Model file for the job. Use its own axes, mm. Face numbers are marked on the shaded views. A direction names the side the tool comes from. Round coordinates to 2 decimals unless told otherwise and drop trailing zeros. One line per item, written item: value.
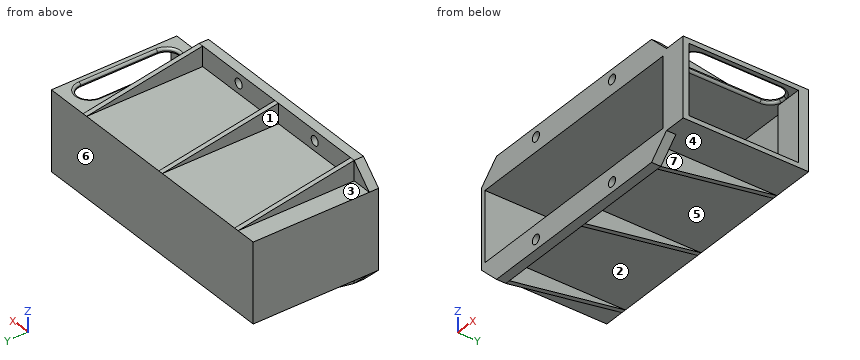
from build123d import *

# Parameters (mm, degrees)
SKETCH1_W                 = 166.85
SKETCH1_H                 = 54.05
SKETCH1_W_2               = 160.5
SKETCH1_H_2               = 47.7
BOSS_EXTRUDE1_DEPTH       = 3.81
BOSS_EXTRUDE2_DEPTH       = 78.232
SKETCH3_W                 = 166.85
SKETCH3_H                 = 54.05
BOSS_EXTRUDE5_DEPTH       = 3.175
SKETCH4_W                 = 3.175
SKETCH4_H                 = 54.05
BOSS_EXTRUDE6_DEPTH       = 3.81
BOSS_EXTRUDE7_DEPTH       = 6.35
BOSS_EXTRUDE9_DEPTH       = 3.175
BOSS_EXTRUDE10_DEPTH      = 3.175
SKETCH8_R                 = 3.175
CUT_EXTRUDE1_DEPTH        = 122.77066278
BOSS_EXTRUDE11_DEPTH      = 1.5875
BOSS_EXTRUDE11_DEPTH_BACK = 1.5875
SKETCH14_W                = 54.05
SKETCH14_H                = 85.217
SKETCH14_W_2              = 47.7
SKETCH14_H_2              = 74.422
BOSS_EXTRUDE13_DEPTH      = 14.986
CUT_EXTRUDE2_DEPTH        = 147.696293869
SKETCH16_W                = 160.5
SKETCH16_H                = 47.7
CUT_EXTRUDE3_DEPTH        = 1.5875
SKETCH17_W                = 18.712657602
SKETCH17_H                = 69.277031054
BOSS_EXTRUDE14_DEPTH      = 3.175
FILLET1_R                 = 1.5875


with BuildPart() as part:
    # Sketch1 → Boss-Extrude1 (new body)
    with BuildSketch(Plane(origin=(0, 0, 0), x_dir=(1, 0, 0), z_dir=(0, 1, 0))):
        Rectangle(SKETCH1_W, SKETCH1_H)
        Rectangle(SKETCH1_W_2, SKETCH1_H_2, mode=Mode.SUBTRACT)
    extrude(amount=BOSS_EXTRUDE1_DEPTH)

    # Sketch2 → Boss-Extrude2 (add)
    with BuildSketch(Plane(origin=(0, 3.81, 0), x_dir=(1, 0, 0), z_dir=(0, 1, 0))):
        Polygon((-83.425, 27.025), (83.425, 27.025), (83.425, 23.85), (80.25, 23.85), (-80.25, 23.85), (-80.25, -23.85), (80.25, -23.85), (83.425, -23.85), (83.425, -27.025), (-83.425, -27.025), align=None)
    extrude(amount=BOSS_EXTRUDE2_DEPTH)

    # Sketch3 → Boss-Extrude5 (add)
    with BuildSketch(Plane(origin=(0, 82.042, 0), x_dir=(1, 0, 0), z_dir=(0, 1, 0))):
        Rectangle(SKETCH3_W, SKETCH3_H)
    extrude(amount=BOSS_EXTRUDE5_DEPTH)

    # Sketch4 → Boss-Extrude6 (add)
    with BuildSketch(Plane.XZ.offset(-82.042)):
        with Locations((81.8375, 0)):
            Rectangle(SKETCH4_W, SKETCH4_H)
    extrude(amount=BOSS_EXTRUDE6_DEPTH)

    # Sketch5 → Boss-Extrude7 (add)
    with BuildSketch(Plane(origin=(0, 0, 0), x_dir=(1, 0, 0), z_dir=(0, 1, 0))):
        Polygon((-83.425, -27.025), (83.425, -27.025), (69.85, -40.6), (-69.85, -40.6), align=None)
        Polygon((-69.85, 40.6), (-83.425, 27.025), (83.425, 27.025), (69.85, 40.6), align=None)
    extrude(amount=BOSS_EXTRUDE7_DEPTH)

    # Sketch6 → Boss-Extrude9 (add)
    with BuildSketch(Plane.ZY.offset(69.85)):
        Polygon((27.025, 85.217), (27.025, 6.35), (40.6, 6.35), align=None)
        Polygon((-27.025, 85.217), (-40.6, 6.35), (-27.025, 6.35), align=None)
    extrude(amount=-BOSS_EXTRUDE9_DEPTH)

    # Sketch7 → Boss-Extrude10 (add)
    with BuildSketch(Plane(origin=(69.85, 0, 0), x_dir=(0, 0, -1), z_dir=(1, 0, 0))):
        Polygon((-27.025, 85.217), (-27.025, 6.35), (-40.6, 6.35), align=None)
        Polygon((40.6, 6.35), (27.025, 85.217), (27.025, 6.35), align=None)
    extrude(amount=-BOSS_EXTRUDE10_DEPTH)

    # Sketch8 → Cut-Extrude1 (cut, through all)
    with BuildSketch(Plane(origin=(0, 6.35, 0), x_dir=(1, 0, 0), z_dir=(0, 1, 0))):
        with Locations(Location((-34.29, -33.812500014, 0), (0, 0, 270))):
            Circle(SKETCH8_R)
        with Locations(Location((34.29, -33.812500014, 0), (0, 0, 90))):
            Circle(SKETCH8_R)
        with Locations(Location((34.29, 33.812500014, 0), (0, 0, 270))):
            Circle(SKETCH8_R)
        with Locations(Location((-34.29, 33.812500014, 0), (0, 0, 90))):
            Circle(SKETCH8_R)
    extrude(amount=-CUT_EXTRUDE1_DEPTH, mode=Mode.SUBTRACT)

    # Sketch11 → Boss-Extrude11 (add, two sides: drawn at the far end of the back side and taken through both)
    with BuildSketch(Plane(origin=(0, 0, 0), x_dir=(0, 0, -1), z_dir=(1, 0, 0)).offset(-BOSS_EXTRUDE11_DEPTH_BACK)):
        Polygon((-27.025, 85.217), (-27.025, 6.35), (-40.6, 6.35), align=None)
        Polygon((40.6, 6.35), (27.025, 85.217), (27.025, 6.35), align=None)
    extrude(amount=BOSS_EXTRUDE11_DEPTH + BOSS_EXTRUDE11_DEPTH_BACK)

    # Sketch14 → Boss-Extrude13 (add)
    with BuildSketch(Plane(origin=(98.411, 0, 0), x_dir=(0, 0, -1), z_dir=(1, 0, 0))):
        with Locations((0, 42.6085)):
            Rectangle(SKETCH14_W, SKETCH14_H)
        with Locations((0, 41.021)):
            Rectangle(SKETCH14_W_2, SKETCH14_H_2, mode=Mode.SUBTRACT)
    extrude(amount=-BOSS_EXTRUDE13_DEPTH)

    # Sketch15 → Cut-Extrude2 (cut, through all)
    with BuildSketch(Plane(origin=(0, 0, -27.025), x_dir=(-1, 0, 0), z_dir=(0, 0, -1))):
        with BuildLine():
            Line((-93.966, 68.707), (-93.966, 16.51))
            ThreePointArc((-93.966, 16.51), (-85.711, 8.255), (-77.456, 16.51))
            Line((-77.456, 16.51), (-77.456, 68.707))
            ThreePointArc((-77.456, 68.707), (-85.711, 76.962), (-93.966, 68.707))
        make_face()
    extrude(amount=-CUT_EXTRUDE2_DEPTH, mode=Mode.SUBTRACT)

    # Sketch16 → Cut-Extrude3 (cut)
    with BuildSketch(Plane.XZ.offset(-82.042)):
        Rectangle(SKETCH16_W, SKETCH16_H)
    extrude(amount=-CUT_EXTRUDE3_DEPTH, mode=Mode.SUBTRACT)

    # Sketch17 → Boss-Extrude14 (add)
    with BuildSketch(Plane(origin=(0, 0, -27.025), x_dir=(-1, 0, 0), z_dir=(0, 0, -1))):
        with Locations((-85.711, 42.6085)):
            Rectangle(SKETCH17_W, SKETCH17_H)
    extrude(amount=-BOSS_EXTRUDE14_DEPTH)

    # Fillet1
    fillet1_edges = [part.edges().sort_by_distance(p)[0] for p in [
        (85.711, 8.255, 23.85),
        (93.966, 42.6085, 23.85),
        (85.711, 76.962, 23.85),
        (85.711, 76.962, 27.025),
        (77.456, 42.6085, 27.025),
        (85.711, 8.255, 27.025),
        (77.456, 42.6085, 23.85),
        (93.966, 42.6085, 27.025),
    ]]
    fillet(fillet1_edges, radius=FILLET1_R - 0.0001)  # a hair under: the kernel refuses the full size


solid = part.part
1. Wall check: probe 1 along Z at (x, y) = (34, 2); probe 2 along Z at (x, y) = (36, 35) (3 decimals); probe 3 along X at (y, z) = (63, -7) (3 decimals). Give the ranges that are in metal, low to high. Write a range as [from, to].
Report:
probe 1: [-40.6, -36.97], [-30.65, -23.85], [23.85, 30.65], [36.97, 40.6]
probe 2: [-27.025, -23.85], [23.85, 27.025]
probe 3: [-83.425, -80.25]
2. Drop flat-ended pins along their axis: pin 1 (1.5 mm diameter, centred on x = 72.5, y = 58, fed in from -Z) (3 decimals); pin 2 (4 mm diameter, centred on x = -7.5, y = 27, fed in from +Z) (3 decimals); pin 3 (2 mm diameter, centred on y = 72, z = -21, fed in from +X); pin 4 (4 mm diameter, centred on x = -34.29, z = 33.81, fed in from +Y). Give the stop position or say it passes through.
Report:
pin 1: z = -27.025
pin 2: z = 27.025
pin 3: x = -80.25
pin 4: through
3. Mould opens along X. For the marked faces 5, 6 and 7 say: released by +X, released by -X, zero draft, split by the parting line, or undercut.
Report:
face 5: undercut
face 6: zero draft
face 7: released by +X
4. Band-saw the part on B-B on x = -34.29. State how many separate pieces and enclosed holes the cut face has, plus the area to 3 significant figures.
Report:
separate pieces: 3
enclosed holes: 0
area: 709 mm²
5. Tool access for the marked faces 1, 2, 3 and 4: list every direction of +Z, -Z, +X, -X, +Y, -Y with a clear straight run to the whole face (end or side of a thin tool).
Report:
face 1: +Z, +Y
face 2: -Z, +Y
face 3: +Z, -X, +Y
face 4: -Z, +X, +Y
